Verification items for this drawing (mm, ordinates from the low corner). Give positions to 0.01 mm unless a question says otherwise; leave off trailing zeros. Loops run counter-clockwise (first coordinate to the right, second up) from the corner with the lowest first, then second, coordinate; pieces in that order, holes last. Notation, with made-up numbers: M 20.5,66.25 L 64.5,66.25 A25 ccw 64.5,103.25 Z; hole C 41,67 d11. An arc over 180 degrees is marked long. Use one line per item in the form item = value.
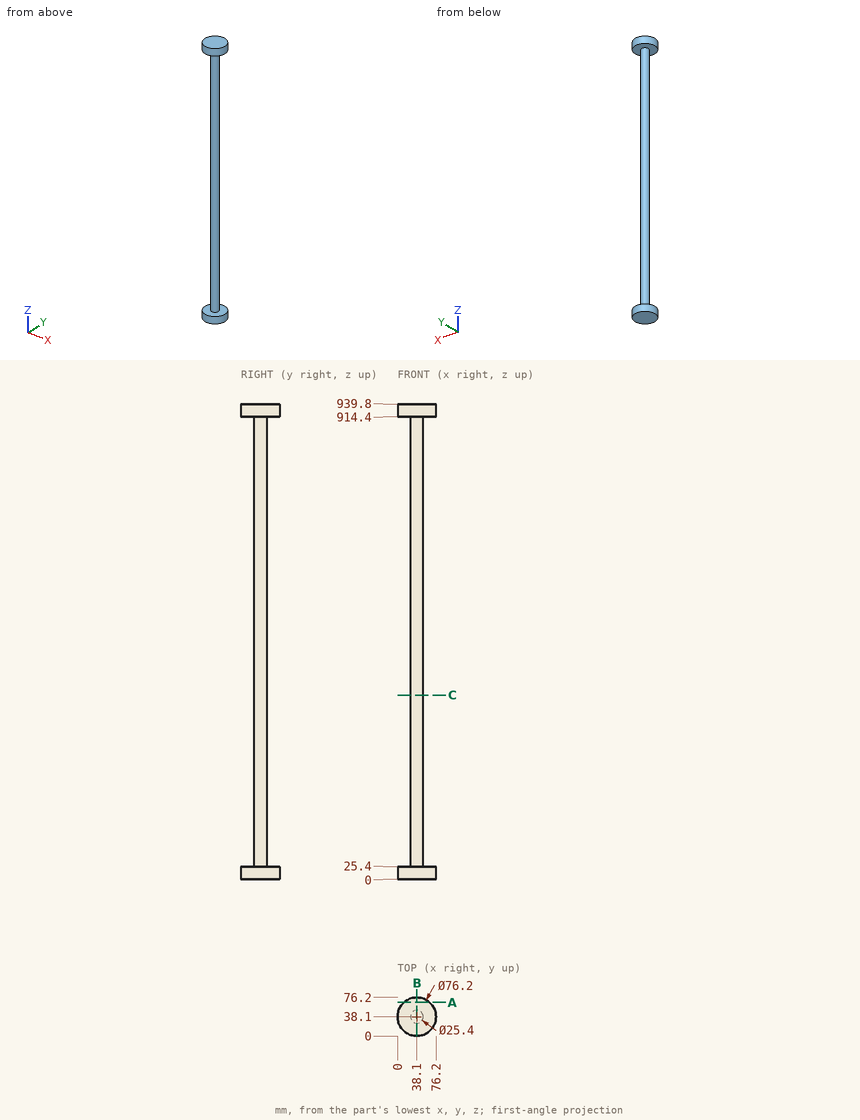
1) Section check B-B (x = 38.1). Record the cut outline in (y, z).
Evaluation:
outline = M 0,0 L 76.2,0 L 76.2,25.4 L 50.8,25.4 L 50.8,914.4 L 76.2,914.4 L 76.2,939.8 L 0,939.8 L 0,914.4 L 25.4,914.4 L 25.4,25.4 L 0,25.4 Z
2) Section check A-A (y = 66.5). Record the cut outline in (x, z), then the cut area to 3 significant figures.
Evaluation:
outline = M 12.7,0 L 63.5,0 L 63.5,25.4 L 12.7,25.4 Z; M 12.7,914.4 L 63.5,914.4 L 63.5,939.8 L 12.7,939.8 Z
area = 2,580 mm^2
3) Depth check by flat-ended pin: pin 1 Ø6 at (x, z) = (40, 796) entering from -Y; pin 2 Ø1 at (x, y) = (36, 10.5) entering from -Z; pin 3 Ø6 at (x, z) = (49.5, 527) entering from +Y; pin 4 Ø1 at (x, z) = (26, 426.5) entering from +Y. Enter the tip coordinate at first touch or a pass-through.
Evaluation:
pin_1 = 25.4
pin_2 = 0
pin_3 = 47.63
pin_4 = 43.27
4) Scan lines: line 1 (Z direction, x = 27.5, y = 54); line 2 (X direction, y = 39, z = 725); line 3 (X direction, y = 40, z = 423.5). Record each from-to range of solid material in increasing order.
Evaluation:
line_1 = 0 to 25.4, 914.4 to 939.8
line_2 = 25.43 to 50.77
line_3 = 25.54 to 50.66
5) Section check C-C (z = 364.5). Record the cut outline in (x, y).
Evaluation:
outline = C 38.1,38.1 d25.4
